Here's how the part is built. I have some questions about the finished solid (model axes, mm). Face numbers are marked on the shaded views. A direction names the side the tool comes from. Give positions to 0.01 mm unless a question says otherwise; leave off trailing zeros. Answer as CSV lines item,"result". Start each with the question number.
Q1. For pin 1 (1.3 mm diameter, centred on x = -4.5, z = 2.5, fed in from +Y); pin 2 (1 mm diameter, centred on y = 1, z = 3.5, fed in from -X), each with a flat end and sliding along its axis, tell me the tip position at first contact or that it passes through.
Q2. If I drill on line 1 along X through (y, z) = (-1.25, 2.75); line 2 along Y through (x, z) = (-11, 1.85); line 3 along Y through (x, z) = (-3, 4.3), over which ranges is the centre line in solid material (lowest first)?
Q3. On a 3-axis mill with a long thin cutter (end or side, diameter ignored), from which of +Z, -Z, +X, -X, +Y, -Y can I reach the whole of each face in a straight line? I mean the marked faces 1 and 2. Say none if no direction works.
Q4. Suppose I cut it at A-A (z = 1.1). Count the separate pieces of the cut face and the enclosed holes in it, then the cut area to 3 significant figures.
```python
from build123d import *

# Parameters (mm, degrees)
SKETCH1_R           = 5
SKETCH1_R_2         = 1.75
BOSS_EXTRUDE1_DEPTH = 4.5
BOSS_EXTRUDE2_START = -4.5
BOSS_EXTRUDE2_DEPTH = 4.5


with BuildPart() as part:
    # Sketch1 → Boss-Extrude1 (new body)
    # profile 1 of 3: a face of its own
    with BuildSketch(Plane.XY):
        with Locations((-11, 0)):
            Circle(SKETCH1_R)
        with Locations((-11, 0)):
            Circle(SKETCH1_R_2, mode=Mode.SUBTRACT)
    # profile 2 of 3: a face of its own
    with BuildSketch(Plane.XY):
        with Locations((11, 0)):
            Circle(SKETCH1_R)
        with Locations((11, 0)):
            Circle(SKETCH1_R_2, mode=Mode.SUBTRACT)
    # profile 3 of 3: a face of its own
    with BuildSketch(Plane.XY):
        with BuildLine():
            Line((11.000000039, 5), (-11, 5))
            ThreePointArc((-11, 5), (-7.464466094, 3.535533906), (-6, 0))
            ThreePointArc((-6, 0), (-7.464466094, -3.535533906), (-11, -5))
            Line((-11, -5), (10.999999969, -5))
            ThreePointArc((10.999999969, -5), (6, 3.5e-08), (11.000000039, 5))
        make_face()
    extrude(amount=BOSS_EXTRUDE1_DEPTH)

    # Sketch2 → Boss-Extrude2 (add)
    with BuildSketch(Plane.XY.offset(4.5).offset(BOSS_EXTRUDE2_START)):
        with BuildLine():
            Line((46.363989199, 12.87), (49.180795902, 10.03))
            Line((49.180795902, 10.03), (42.27, 6))
            add(Edge.make_bspline(
                [(42.27, 6), (33.457840426, 7.213673904), (27.801569406, 2.343916059), (20.61, -1.48)],
                knots=[0, 0, 0, 0, 1, 1, 1, 1], degree=3))
            Line((20.61, -1.48), (13.99, -5))
            Line((13.99, -5), (11, -5))
            ThreePointArc((11, -5), (16, 0), (11, 5))
            Line((11, 5), (0, 5))
            add(Edge.make_bspline(
                [(0, 5), (22.387497142, 13.115081385), (46.363989199, 12.87)],
                knots=[0, 0, 0, 1, 1, 1], degree=2))
        make_face()
    extrude(amount=BOSS_EXTRUDE2_DEPTH)


solid = part.part
```
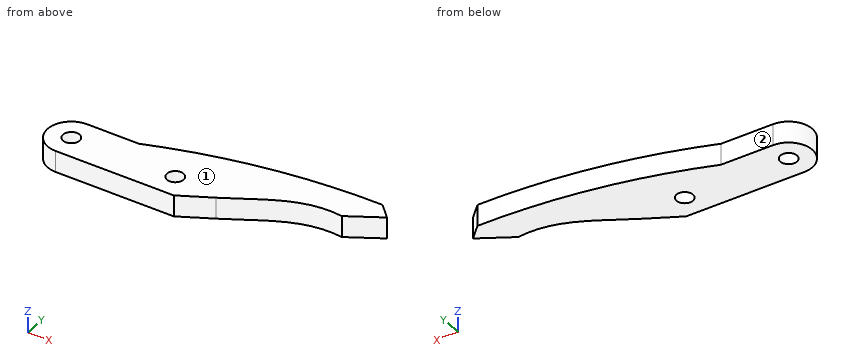
Resolved:
1,pin 1,"y = 5"
1,pin 2,"x = -15.97"
2,line 1,"-15.84 to -12.22, -9.78 to 9.78, 12.22 to 21.04"
2,line 2,"-5 to -1.75, 1.75 to 5"
2,line 3,"-5 to 5"
3,face 1,"+Z, +X, -X, +Y, -Y"
3,face 2,"+Z, -Z, -X, +Y"
4,separate pieces,"1"
4,enclosed holes,"2"
4,area,"600 mm^2"
